Input: part model. Units: mm. Frame: model coordinates. Coordinates: 2 decimals unless noted, no trailing zeros. Order: outer loops, then holes, each group sorted by start corner. A loop starts at its lowest first (then second) coordinate and runs counter-clockwise, first axis right, second up. Notation, with made-up numbers: (-37, 2) - (-2, 2) arc R3 ccw to (-2, 6) - close; hole circle Ø6 at (-5, 74). An arc over 180 degrees is marked (long way). Answer as CSV lines item,"result". Start each with the question number.
Item 1: Section B-B (x = -19.5). Output: boundary loops of the cut face in (y, z), and give its area (3 significant figures).
Item 2: Section A-A (z = 15). Output: boundary loops of the cut face in (x, y), and give its area (3 significant figures).
Item 3: Material intervals for line 1 along X through (y, z) = (3.75, -5); line 2 along Z through (x, y) = (-19.5, 1.35); line 3 along X through (y, z) = (2.7, 15), sorted ascending.
Item 4: Section C-C (z = -15). Output: boundary loops of the cut face in (x, y), and give its area (3 significant figures).
Item 5: Section D-D (z = 47). Output: boundary loops of the cut face in (x, y).
Item 6: First-contact query: pin 1 (1.5 mm diameter, centred on x = 1.5, y = 0.5, fed in from +Z); pin 2 (0.6 mm diameter, centred on x = 3, y = 1.5, fed in from -Z). Flat tips, straight axial feed; report the tip coordinate or a pass-through.
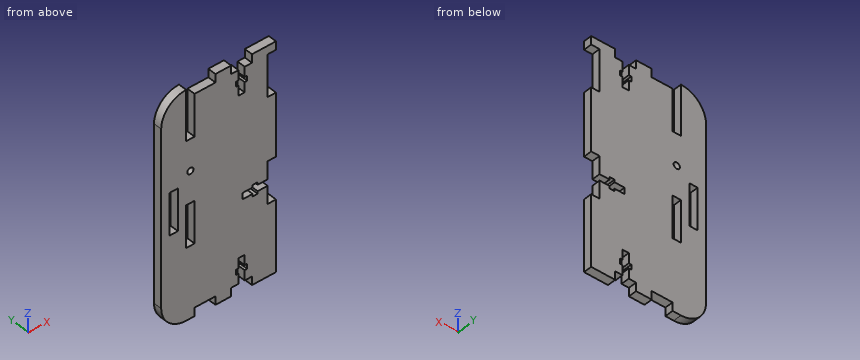
Autodesk Inventor part; units mm, degrees
ref_plane "YZ Plane" through (0, 0, 0) normal (1, 0, 0) x (0, 1, 0)
ref_plane "XZ Plane" through (0, 0, 0) normal (0, 1, 0) x (-1, 0, 0)
ref_plane "XY Plane" through (0, 0, 0) normal (0, 0, 1) x (1, 0, 0)
sketch "Sketch1" plane through (0, 0, 0) normal (0, 1, 0) x (-1, 0, 0)
  line L0 (-17.5, 50) -> (17.5, 50)
  line L1 (17.5, 50) -> (17.5, -50)
  line L2 (17.5, -50) -> (-17.5, -50)
  line L3 (-17.5, -50) -> (-17.5, 50)
  line L4 (-17.5, 50) -> (17.5, -50) construction
  line L5 (17.5, 50) -> (-17.5, -50) construction
  line L6 (7.5, 50) -> (0, 50)
  line L7 (0, 50) -> (0, 54)
  line L8 (0, 54) -> (7.5, 54)
  line L9 (7.5, 54) -> (7.5, 50)
  line L10 (-10, 50) -> (-21.5, 50)
  line L11 (-21.5, 50) -> (-21.5, 54)
  line L12 (-21.5, 54) -> (-10, 54)
  line L13 (-10, 54) -> (-10, 50)
  line L14 (17.5, 30) -> (21.5, 30)
  line L15 (21.5, 30) -> (21.5, 0)
  line L16 (21.5, 0) -> (17.5, 0)
  line L17 (17.5, 0) -> (17.5, 30)
  line L18 (17.5, -20) -> (21.5, -20)
  line L19 (21.5, -20) -> (21.5, -54)
  line L20 (21.5, -54) -> (17.5, -54)
  line L21 (17.5, -54) -> (17.5, -20)
  line L22 (7.5, -50) -> (0, -50)
  line L23 (0, -50) -> (0, -54)
  line L24 (0, -54) -> (7.5, -54)
  line L25 (7.5, -54) -> (7.5, -50)
  line L26 (-10, -50) -> (-21.5, -50)
  line L27 (-21.5, -50) -> (-21.5, -54)
  line L28 (-21.5, -54) -> (-10, -54)
  line L29 (-10, -54) -> (-10, -50)
  line L30 (-17.5, 30) -> (-21.5, 30)
  line L31 (-21.5, 30) -> (-21.5, 0)
  line L32 (-21.5, 0) -> (-17.5, 0)
  line L33 (-17.5, 0) -> (-17.5, 30)
  line L34 (-17.5, -50) -> (-21.5, -50)
  line L35 (-21.5, -50) -> (-21.5, -20)
  line L36 (-21.5, -20) -> (-17.5, -20)
  line L37 (-17.5, -20) -> (-17.5, -50)
  point P0 (0, 0)
  point P1 (17.5, 0)
  point P2 (-17.5, 50)
  point P3 (-17.5, 0)
  point P4 (-21.5, -50)
  point P5 (17.5, -50)
  point P6 (19.5, -54)
  dimension "d0" = 35
  dimension "d2" = 7.5
  dimension "d3" = 4
  dimension "d4" = 11.5
  dimension "d5" = 4
  dimension "d6" = 10
  dimension "d7" = 10
  dimension "d8" = 4
  dimension "d9" = 30
  dimension "d10" = 4
  dimension "d11" = 34
  dimension "d12" = 20
  dimension "d13" = 20
  dimension "d14" = 7.5
  dimension "d15" = 4
  dimension "d16" = 11.5
  dimension "d17" = 4
  dimension "d18" = 10
  dimension "d19" = 10
  dimension "d20" = 4
  dimension "d21" = 30
  dimension "d22" = 20
  dimension "d23" = 4
  dimension "d24" = 30
  dimension "d27" = 4
extrude "Extrusion1" add sketch "Sketch1" along normal blind 4
sketch "Sketch2" plane through (0, 4, 0) normal (0, 1, 0) x (1, 0, 0)
  line L0 (-21.5, 54) -> (-33.5, 54)
  line L1 (-33.5, 54) -> (-33.5, -54)
  line L2 (-33.5, -54) -> (-21.5, -54)
  line L3 (-21.5, -54) -> (-21.5, 54)
  line L4 (-21.5, 54) -> (-21.5, 20)
  line L5 (-21.5, 20) -> (-17.5, 20)
  line L6 (-17.5, 20) -> (-17.5, 0)
  line L7 (-17.5, 0) -> (-21.5, 0)
  line L8 (-21.5, 0) -> (-21.5, -30)
  line L9 (-21.5, -30) -> (-17.5, -30)
  line L10 (-17.5, -30) -> (-17.5, -50)
  line L11 (-17.5, -50) -> (-7.5, -50)
  line L12 (-7.5, -50) -> (-7.5, -54)
  line L13 (-7.5, -54) -> (0, -54)
  line L14 (0, -54) -> (0, -50)
  line L15 (0, -50) -> (10, -50)
  line L16 (10, -50) -> (10, -54)
  line L17 (10, -54) -> (21.5, -54)
  line L18 (21.5, -54) -> (21.5, -50)
  line L19 (21.5, -50) -> (17.5, -50)
  line L20 (17.5, -50) -> (17.5, -30)
  line L21 (17.5, -30) -> (21.5, -30)
  line L22 (21.5, -30) -> (21.5, 0)
  line L23 (21.5, 0) -> (17.5, 0)
  line L24 (17.5, 0) -> (17.5, 20)
  line L25 (17.5, 20) -> (21.5, 20)
  line L26 (21.5, 20) -> (21.5, 54)
  line L27 (21.5, 54) -> (10, 54)
  line L28 (10, 54) -> (10, 50)
  line L29 (10, 50) -> (0, 50)
  line L30 (0, 50) -> (0, 54)
  line L31 (0, 54) -> (-7.5, 54)
  line L32 (-7.5, 54) -> (-7.5, 50)
  line L33 (-7.5, 50) -> (-17.5, 50)
  line L34 (-17.5, 50) -> (-17.5, 54)
  line L35 (-17.5, 54) -> (-21.5, 54)
  line L36 (-7.5, -54) -> (0, -54)
  line L37 (-33.5, 54) -> (21.5, -54) construction
  line L38 (-29.5, 10) -> (-25.5, 10)
  line L39 (-25.5, 10) -> (-25.5, -10)
  line L40 (-25.5, -10) -> (-29.5, -10)
  line L41 (-29.5, -10) -> (-29.5, 10)
  point P0 (0, 0)
  point P1 (-6, 0)
  point P2 (-25.5, 0)
  dimension "d28" = 51
  dimension "d34" = 20
  dimension "d35" = 4
  dimension "d36" = 4
extrude "Extrusion2" add sketch "Sketch2" against normal up to surface (4 mm away) contours L3 L2 L1 L0
sketch "Sketch3" plane through (0, 4, 0) normal (0, 1, 0) x (1, 0, 0)
  line L0 (3.5, 45.2) -> (3.5, 50)
  line L1 (3.5, 50) -> (0, 50)
  line L2 (0, 50) -> (0, 54) construction
  line L3 (0, 54) -> (-7.5, 54) construction
  line L4 (-7.5, 54) -> (-7.5, 50) construction
  line L5 (-7.5, 50) -> (-17.5, 50) construction
  line L6 (-17.5, 50) -> (-17.5, 54) construction
  line L7 (-17.5, 54) -> (-21.5, 54) construction
  line L8 (-17.5, 0) -> (-21.5, 0) construction
  line L9 (-21.5, 0) -> (-21.5, -30) construction
  line L10 (-21.5, -30) -> (-17.5, -30) construction
  line L11 (-17.5, -30) -> (-17.5, -50) construction
  line L12 (-17.5, -50) -> (-7.5, -50) construction
  line L13 (-7.5, -50) -> (-7.5, -54) construction
  line L14 (-7.5, -54) -> (0, -54) construction
  line L15 (0, -54) -> (0, -50) construction
  line L16 (0, -50) -> (3.5, -50)
  line L17 (3.5, -50) -> (3.5, -45.2)
  line L18 (3.5, -45.2) -> (2.3, -45.2)
  line L19 (2.3, -45.2) -> (2.3, -42.8)
  line L20 (2.3, -42.8) -> (3.5, -42.8)
  line L21 (3.5, -42.8) -> (3.5, -38)
  line L22 (3.5, -38) -> (6.5, -38)
  line L23 (6.5, -38) -> (6.5, -42.8)
  line L24 (6.5, -42.8) -> (7.7, -42.8)
  line L25 (7.7, -42.8) -> (7.7, -45.2)
  line L26 (7.7, -45.2) -> (6.5, -45.2)
  line L27 (6.5, -45.2) -> (6.5, -50)
  line L28 (6.5, -50) -> (10, -50) construction
  line L29 (10, -50) -> (10, -54) construction
  line L30 (10, -54) -> (21.5, -54) construction
  line L31 (21.5, -54) -> (21.5, -50) construction
  line L32 (21.5, -50) -> (17.5, -50) construction
  line L33 (17.5, -50) -> (17.5, -30) construction
  line L34 (17.5, -30) -> (21.5, -30) construction
  line L35 (21.5, 0) -> (17.5, 0) construction
  line L36 (17.5, 0) -> (17.5, 8.5) construction
  line L37 (17.5, 8.5) -> (12.7, 8.5)
  line L38 (12.7, 8.5) -> (12.7, 7.3)
  line L39 (12.7, 7.3) -> (10.3, 7.3)
  line L40 (10.3, 7.3) -> (10.3, 8.5)
  line L41 (10.3, 8.5) -> (5.5, 8.5)
  line L42 (5.5, 8.5) -> (5.5, 11.5)
  line L43 (5.5, 11.5) -> (10.3, 11.5)
  line L44 (10.3, 11.5) -> (10.3, 12.7)
  line L45 (10.3, 12.7) -> (12.7, 12.7)
  line L46 (12.7, 12.7) -> (12.7, 11.5)
  line L47 (12.7, 11.5) -> (17.5, 11.5)
  line L48 (17.5, 11.5) -> (17.5, 20) construction
  line L49 (17.5, 20) -> (21.5, 20) construction
  line L50 (21.5, 20) -> (21.5, 54) construction
  line L51 (21.5, 54) -> (10, 54) construction
  line L52 (10, 54) -> (10, 50) construction
  line L53 (10, 50) -> (6.5, 50)
  line L54 (6.5, 50) -> (6.5, 45.2)
  line L55 (6.5, 45.2) -> (7.7, 45.2)
  line L56 (7.7, 45.2) -> (7.7, 42.8)
  line L57 (7.7, 42.8) -> (6.5, 42.8)
  line L58 (6.5, 42.8) -> (6.5, 38)
  line L59 (6.5, 38) -> (3.5, 38)
  line L60 (3.5, 38) -> (3.5, 42.8)
  line L61 (3.5, 42.8) -> (2.3, 42.8)
  line L62 (2.3, 42.8) -> (2.3, 45.2)
  line L63 (2.3, 45.2) -> (3.5, 45.2)
  circle A0 centre (-19.5, -15) radius 1.5
  line L64 (-21.5, -30) -> (-17.5, -30) construction
  line L65 (-17.5, -30) -> (-17.5, -50) construction
  line L66 (-17.5, -50) -> (-7.5, -50) construction
  line L67 (-7.5, -50) -> (-7.5, -54) construction
  line L68 (-7.5, -54) -> (0, -54) construction
  line L69 (0, -54) -> (0, -50) construction
  line L70 (0, -50) -> (10, -50)
  line L71 (10, -50) -> (10, -54) construction
  line L72 (10, -54) -> (21.5, -54) construction
  line L73 (21.5, -54) -> (21.5, -50) construction
  line L74 (21.5, -50) -> (17.5, -50) construction
  line L75 (17.5, -50) -> (17.5, -30) construction
  line L76 (17.5, -30) -> (21.5, -30) construction
  line L77 (21.5, -30) -> (21.5, 0) construction
  line L78 (21.5, 0) -> (17.5, 0) construction
  line L79 (17.5, 0) -> (17.5, 20)
  line L80 (17.5, 20) -> (21.5, 20) construction
  line L81 (21.5, 20) -> (21.5, 54) construction
  line L82 (21.5, 54) -> (10, 54) construction
  line L83 (10, 54) -> (10, 50) construction
  line L84 (10, 50) -> (0, 50)
  line L85 (0, 50) -> (0, 54) construction
  line L86 (0, 54) -> (-7.5, 54) construction
  line L87 (-7.5, 54) -> (-7.5, 50) construction
  line L88 (-7.5, 50) -> (-17.5, 50) construction
  line L89 (-17.5, 50) -> (-17.5, 54) construction
  line L90 (-17.5, 54) -> (-33.5, 54) construction
  line L91 (-33.5, 54) -> (-33.5, -54) construction
  line L92 (-33.5, -54) -> (-21.5, -54) construction
  line L93 (-21.5, -54) -> (-21.5, -30) construction
  line L94 (-29.5, 10) -> (-25.5, 10) construction
  line L95 (-25.5, 10) -> (-25.5, -10) construction
  line L96 (-25.5, -10) -> (-29.5, -10) construction
  line L97 (-29.5, -10) -> (-29.5, 10) construction
  line L98 (-21.5, 0) -> (-21.5, 20) construction
  line L99 (-21.5, 20) -> (-17.5, 20) construction
  line L100 (-17.5, 20) -> (-17.5, 0)
  line L101 (-17.5, 0) -> (-21.5, 0) construction
  point P0 (0, 0)
  point P1 (-17.5, 11.5)
  point P2 (-12.7, 8.5)
extrude "Extrusion3" cut sketch "Sketch3" against normal up to next
fillet "Fillet1" radius 12 2 edges at (-33.5, 2, 54) (-33.5, 2, -54)
properties part number "FloorButtonHolder_Bottom_V1_B" material "MDF Medium Density Fiberboard"
Determined:
1,outline,"(0, -54) - (4, -54) - (4, -20) - (0, -20) - close; (0, 0) - (4, 0) - (4, 13.5) - (0, 13.5) - close; (0, 16.5) - (4, 16.5) - (4, 30) - (0, 30) - close"
1,area,"244 mm^2"
2,outline,"(-33.5, 0) - (-21, 0) - (-21, 4) - (-33.5, 4) - close; (-18, 0) - (21.5, 0) - (21.5, 4) - (-18, 4) - close"
2,area,"208 mm^2"
3,line 1,"x = -33.5 to -29.5, -25.5 to -21.5, -17.5 to 17.5"
3,line 2,"z = -54 to -20, 0 to 13.5, 16.5 to 30"
3,line 3,"x = -33.5 to -21, -18 to 21.5"
4,outline,"(-33.5, 0) - (-21.5, 0) - (-21.5, 4) - (-33.5, 4) - close; (-17.5, 0) - (17.5, 0) - (17.5, 4) - (-17.5, 4) - close"
4,area,"188 mm^2"
5,outline,"(-32.41, 0) - (-21.5, 0) - (-21.5, 4) - (-32.41, 4) - close; (-17.5, 0) - (3.5, 0) - (3.5, 4) - (-17.5, 4) - close; (6.5, 0) - (17.5, 0) - (17.5, 4) - (6.5, 4) - close"
6,pin 1,"stops at z = 50"
6,pin 2,"stops at z = -50"
